Input: part model. Units: mm. Frame: model coordinates. Coordinates: 2 decimals unless noted, no trailing zeros. Write each loop counter-clockwise with the first axis right and the second up, starting at its lowest first coordinate (ties: lowest second). Pieces come first, ordered by that corner, then holes. Notation, with made-up numbers: M 60,75.5 L 105,75.5 A28 cw 105,113.5 Z; hole C 74.5,20 d9. An arc over 180 degrees is marked long. Write each question's results on one line, items separated by ' | '. Start each with the question number.
1. Ray query, probe 1 along X at (y, z) = (1.25, 11.5); probe 2 along X at (y, z) = (0.75, -10.5); probe 3 along Z at (x, y) = (0, 2.15). Return the intervals inside material, ascending.
2. Section query B-B, the plane z = -70. Output: boundary loops of the cut face in (x, y), and give its area (3 significant figures).
3. Section query D-D, the plane z = -47.1. Output: boundary loops of the cut face in (x, y).
4. Section query A-A, the plane z = 2. Output: boundary loops of the cut face in (x, y), and give its area (3 significant figures).
5. Section query C-C, the plane y = 1.85. Count the separate pieces of the cut face and the enclosed holes in it, and give its area (3 significant figures).
6. First-contact query: pin 1 (1.8 mm diameter, centred on x = 5.91, z = -10, fed in from -Y). Flat tip, straight axial feed; report the tip coordinate or a pass-through.
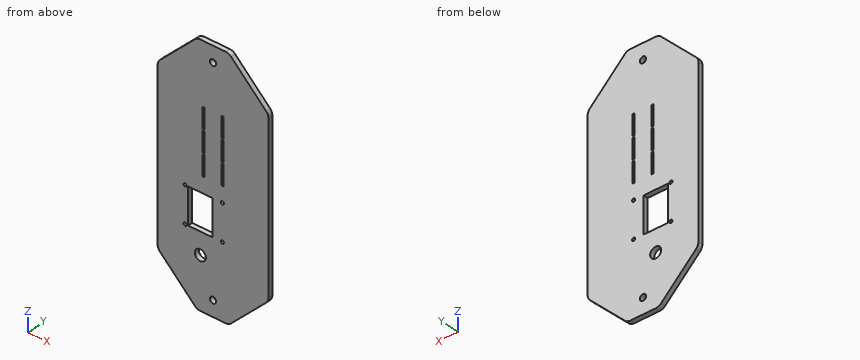
Autodesk Inventor part; units mm, degrees
ref_plane "YZ Plane" through (0, 0, 0) normal (1, 0, 0) x (0, 1, 0)
ref_plane "XZ Plane" through (0, 0, 0) normal (0, 1, 0) x (-1, 0, 0)
ref_plane "XY Plane" through (0, 0, 0) normal (0, 0, 1) x (1, 0, 0)
sketch "Sketch1" plane through (0, 0, 0) normal (0, 1, 0) x (-1, 0, 0)
  line L0 (0, 0) -> (0, 80)
  line L1 (0, 80) -> (0, -80)
  line L2 (0, 80) -> (35, 80)
  line L3 (35, 80) -> (35, -80)
  line L4 (35, -80) -> (-35, -80)
  line L5 (-35, -80) -> (-35, 80)
  line L6 (-35, 80) -> (0, 80)
  line L7 (0, 80) -> (10, 80)
  line L8 (35, 80) -> (35, 55)
  line L9 (10, 80) -> (35, 55)
  line L10 (35, 0) -> (-35, 0)
  line L11 (0, 80) -> (0, -80)
  line L12 (10, -80) -> (35, -55)
  line L13 (-10, 80) -> (-35, 55)
  line L14 (-10, -80) -> (-35, -55)
  line L15 (0, 0) -> (0, 70)
  line L16 (0, 70) -> (0, -70)
  circle A0 centre (0, 70) radius 2
  circle A1 centre (0, -70) radius 2
  dimension "d0" = 80
  dimension "d1" = 160
  dimension "d2" = 35
  dimension "d3" = 70
  dimension "d4" = 10
  dimension "d5" = 25
  dimension "d6" = 70
  dimension "d7" = 140
  dimension "d8" = 4
  dimension "d9" = 4
extrude "Extrusion1" add sketch "Sketch1" along normal blind 3 contours L10 L5 L13 L6 L0 A0 | L10 L3 L12 L4 L1 A1 | L0 A0 L2 L9 L3 L10 | L1 A1 L4 L14 L5 L10
fillet "Fillet1" radius 5 8 edges at (-35, 1.5, 55) (-10, 1.5, 80) (-35, 1.5, -55) (35, 1.5, 55) (10, 1.5, 80) (35, 1.5, -55) (10, 1.5, -80) (-10, 1.5, -80)
sketch "Sketch2" plane through (0, 3, 0) normal (0, 1, 0) x (1, 0, 0)
  line L0 (0, 0) -> (0, 10)
  line L1 (5.9101, 10) -> (-17.6499, 10)
  line L2 (-17.6499, 10) -> (-17.6499, 33.1)
  line L3 (-17.6499, 33.1) -> (5.9101, 33.1)
  line L4 (5.9101, 33.1) -> (5.9101, 10)
  line L5 (0, 10) -> (0, 21.55)
  line L6 (0, 21.55) -> (20, 21.55)
  line L7 (35, -52.9289) -> (35, 52.9289)
  circle A0 centre (20, 21.55) radius 3.5
  circle A1 centre (-17.6499, 10) radius 1
  circle A2 centre (-17.6499, 33.1) radius 1
  circle A3 centre (5.9101, 10) radius 1
  circle A4 centre (5.9101, 33.1) radius 1
  line L8 (0, 0) -> (-6, 0)
  line L9 (-6, 0) -> (-6, -50)
  line L10 (-6, -50) -> (6, -50)
  line L11 (6, -50) -> (6, 0)
  line L12 (6, 0) -> (-6, 0)
  line L13 (-6, -50) -> (-6.5, -50)
  line L14 (-6.5, -50) -> (-6.5, 0)
  line L15 (-6.5, 0) -> (-5.5, 0)
  line L16 (-5.5, 0) -> (-5.5, -50)
  line L17 (-5.5, -50) -> (-6.5, -50)
  line L18 (0, 0) -> (0, -66.8235)
  line L19 (6, -50) -> (6.5, -50)
  line L20 (6.5, -50) -> (6.5, 0)
  line L21 (6.5, 0) -> (5.5, 0)
  line L22 (5.5, 0) -> (5.5, -50)
  line L23 (5.5, -50) -> (6.5, -50)
  line L24 (0, 21.55) -> (6, 21.55)
  dimension "d13" = 10
  dimension "d14" = 23.56
  dimension "d15" = 23.1
  dimension "d16" = 11.55
  dimension "d17" = 20
  dimension "d18" = 7
  dimension "d19" = 2
  dimension "d20" = 2
  dimension "d21" = 2
  dimension "d22" = 2
  dimension "d23" = 6
  dimension "d24" = 50
  dimension "d25" = 12
  dimension "d26" = 0.5
  dimension "d27" = 1
  dimension "d37" = 6
extrude "Extrusion2" cut sketch "Sketch2" against normal blind 10 contours A0 | L16 L10 L9 L8 | L12 L11 L10 L22 | A1 L2 L1 | L1 L2 A1 | A3 L4 L1 | L1 L4 A3 | L9 L13 L14 L15 | L21 L20 L19 L11 | A2 L3 L2 | L2 L3 A2 | A4 L3 L4 | L4 L3 A4
sketch "Sketch3" plane through (0, 3, 0) normal (0, 1, 0) x (1, 0, 0)
  line L0 (-5.5, -50) -> (-5.5, 0)
  line L1 (-5.5, 0) -> (-5.5, -13)
  line L2 (-5.5, -13) -> (-6.5, -13)
  line L3 (-6.5, -50) -> (-6.5, 0)
  line L4 (-6.5, 0) -> (-6.5, -13)
  line L5 (-6.5, 0) -> (-5.5, 0)
  line L6 (-6.5, -13) -> (-6.5, -14)
  line L7 (-6.5, -14) -> (-5.5, -14)
  line L8 (-5.5, -14) -> (-5.5, -13)
  line L9 (-6.5, -13) -> (-5.5, -13)
  line L10 (-6.5, -14) -> (-6.5, -27)
  line L11 (-6.5, -27) -> (-6.5, -28)
  line L12 (-6.5, -28) -> (-5.5, -28)
  line L13 (-5.5, -28) -> (-5.5, -27)
  line L14 (-5.5, -27) -> (-6.5, -27)
  line L15 (-5.5, -14) -> (-5.5, -27)
  line L16 (-6.5, -28) -> (-6.5, -41)
  line L17 (-6.5, -41) -> (-5.5, -41)
  line L18 (-5.5, -41) -> (-5.5, -28)
  line L19 (-6.5, -28) -> (-5.5, -28)
  line L20 (-6.5, -50) -> (-5.5, -50)
  line L21 (-6.5, -41) -> (-6.5, -50)
  line L22 (-6.5, -50) -> (-5.5, -50)
  line L23 (-5.5, -50) -> (-5.5, -41)
  line L24 (0, 0) -> (0, -62.7524)
  line L25 (5.5, -50) -> (5.5, 0)
  line L26 (5.5, -13) -> (6.5, -13)
  line L27 (6.5, -50) -> (6.5, 0)
  line L28 (6.5, 0) -> (5.5, 0)
  line L29 (6.5, -14) -> (5.5, -14)
  line L30 (6.5, -28) -> (5.5, -28)
  line L31 (5.5, -27) -> (6.5, -27)
  line L32 (6.5, -41) -> (5.5, -41)
  line L33 (6.5, -50) -> (5.5, -50)
  dimension "d30" = 13
  dimension "d31" = 1
  dimension "d32" = 13
  dimension "d33" = 1
  dimension "d34" = 13
extrude "Extrusion3" add sketch "Sketch3" against normal blind 3 contours L20 L3 L17 L0 | L12 L3 L14 L0 | L7 L3 L2 L0 | L25 L32 L27 L33 | L25 L31 L27 L30 | L25 L26 L27 L29
sketch "Sketch4" plane through (0, 3, 0) normal (0, 1, 0) x (1, 0, 0)
  circle A0 centre (-17.6499, 10) radius 1
  line L0 (-17.6499, 10) -> (-15.6499, 10)
  circle A1 centre (-17.6499, 33.1) radius 1
  line L1 (-17.6499, 33.1) -> (-15.6499, 33.1)
  line L2 (-15.6499, 10) -> (-15.6499, 33.1)
  circle A2 centre (5.9101, 33.1) radius 1
  line L3 (5.9101, 33.1) -> (-0.3899, 33.1)
  circle A3 centre (5.9101, 10) radius 1
  line L4 (5.9101, 10) -> (-0.3899, 10)
  line L5 (-15.6499, 10) -> (-0.3899, 10)
  line L6 (-0.3899, 10) -> (-0.3899, 33.1)
  line L7 (-0.3899, 33.1) -> (-15.6499, 33.1)
  point P0 (0, 0)
  dimension "d38" = 2
  dimension "d39" = 2
  dimension "d40" = 6.3
  dimension "d41" = 6.3
extrude "Extrusion4" cut sketch "Sketch4" against normal blind 10 contours L2 L7 L6 L5
sketch "Sketch5" plane through (0, 3, 0) normal (0, 1, 0) x (1, 0, 0)
  circle A0 centre (20, 21.55) radius 3.5
  circle A1 centre (20, 21.55) radius 3.5
  point P0 (0, 0)
extrude "Extrusion5" add sketch "Sketch5" against normal blind 3
sketch "Sketch6" plane through (0, 3, 0) normal (0, 1, 0) x (1, 0, 0)
  line L0 (0, 0) -> (0, 62.477)
  line L1 (-15.6499, 33.1) -> (-0.3899, 33.1)
  line L2 (-8.0199, 33.1) -> (-8.0199, 54.1)
  line L3 (-8.0199, 54.1) -> (0, 54.1)
  line L4 (-8.0199, 33.1) -> (-8.0199, 41.1)
  line L5 (-8.0199, 33.1) -> (-8.0199, 47.1)
  circle A0 centre (-8.0199, 47.1) radius 3.5
  dimension "d46" = 21
  dimension "d47" = 8
  dimension "d48" = 14
  dimension "d49" = 7
extrude "Extrusion6" cut sketch "Sketch6" against normal blind 3
properties part number "panel"
Answer:
1) probe 1: -35 to -6.5, -5.5 to 5.5, 6.5 to 35 | probe 2: -35 to -18.52, -16.78 to -15.65, -0.39 to 5.04, 6.78 to 35 | probe 3: -80 to -72, -68 to 68, 72 to 80
2) outline: M -20,0 L -2,0 L -2,3 L -20,3 Z; M 2,0 L 20,0 L 20,3 L 2,3 Z | area: 108 mm^2
3) outline: M -35,0 L -11.52,0 L -11.52,3 L -35,3 Z; M -4.52,0 L 35,0 L 35,3 L -4.52,3 Z
4) outline: M -35,0 L -6.5,0 L -6.5,3 L -35,3 Z; M -5.5,0 L 5.5,0 L 5.5,3 L -5.5,3 Z; M 6.5,0 L 35,0 L 35,3 L 6.5,3 Z | area: 204 mm^2
5) separate pieces: 1 | enclosed holes: 14 | area: 9,440 mm^2
6) pin 1: through
